The model under review builds one solid part; all positions refer to its coordinate system, in mm. A direction names the side the tool comes from. Give positions to 0.01 mm unless a question says otherwise; leave off trailing zeros. Order: outer loops, then holes, each group sorted by start corner. A loop starts at its lowest first (then second) coordinate and runs counter-clockwise, first axis right, second up. Notation, with made-up numbers: (22.5, 14.25) - (56.5, 14.25) arc R20 ccw to (56.5, 19.25) - close; hole circle Ø2 at (45, 70.5). An arc over 180 degrees is marked (long way). Put each result on its own line as item: value.
```python
from build123d import *

# Parameters (mm, degrees)
BOSS_EXTRUDE1_DEPTH = 2
BOSS_EXTRUDE2_DEPTH = 13
SKETCH3_R           = 1.55
CUT_EXTRUDE1_DEPTH  = 16


with BuildPart() as part:
    # Sketch1 → Boss-Extrude1 (new body)
    with BuildSketch(Plane.XY):
        with BuildLine():
            Line((-31.239860577, -6.933333333), (-36, -6.933333333))
            Line((-36, -6.933333333), (-36, 6.933333333))
            Line((-36, 6.933333333), (-31.239860577, 6.933333333))
            ThreePointArc((-31.239860577, 6.933333333), (0, 32), (31.239860577, 6.933333333))
            Line((31.239860577, 6.933333333), (36, 6.933333333))
            Line((36, 6.933333333), (36, -6.933333333))
            Line((36, -6.933333333), (31.239860577, -6.933333333))
            ThreePointArc((31.239860577, -6.933333333), (0, -32), (-31.239860577, -6.933333333))
        make_face()
    extrude(amount=BOSS_EXTRUDE1_DEPTH)

    # Sketch2 → Boss-Extrude2 (add)
    with BuildSketch(Plane.XY.offset(2)):
        with BuildLine():
            Line((-29.428567245, 12.568191195), (-27.589281792, 11.782679245))
            ThreePointArc((-27.589281792, 11.782679245), (0, 30), (27.589281792, 11.782679245))
            Line((27.589281792, 11.782679245), (29.428567245, 12.568191195))
            ThreePointArc((29.428567245, 12.568191195), (0, 32), (-29.428567245, 12.568191195))
        make_face()
        with BuildLine():
            Line((27.589281792, -11.782679245), (29.428567245, -12.568191195))
            ThreePointArc((29.428567245, -12.568191195), (0, -32), (-29.428567245, -12.568191195))
            Line((-29.428567245, -12.568191195), (-27.589281792, -11.782679245))
            ThreePointArc((-27.589281792, -11.782679245), (0, -30), (27.589281792, -11.782679245))
        make_face()
    extrude(amount=BOSS_EXTRUDE2_DEPTH)

    # Sketch3 → Cut-Extrude1 (cut, through all)
    with BuildSketch(Plane(origin=(0, 0, 0), x_dir=(-1, 0, 0), z_dir=(0, 0, -1))):
        with Locations((-33, 0)):
            Circle(SKETCH3_R)
        with Locations((33, 0)):
            Circle(SKETCH3_R)
    extrude(amount=-CUT_EXTRUDE1_DEPTH, mode=Mode.SUBTRACT)


solid = part.part
```
(1) Take a section at D-D, the plane y = 15.5. Write out the cut boundary in (x, z), then the cut area to 3 significant figures.
The answers:
outline: (-28, 0) - (28, 0) - (28, 15) - (25.69, 15) - (25.69, 2) - (-25.69, 2) - (-25.69, 15) - (-28, 15) - close
area: 172 mm^2
(2) Take a section at B-B, the plane x = -33. Write out the cut boundary in (y, z).
The answers:
outline: (-6.93, 0) - (-1.55, 0) - (-1.55, 2) - (-6.93, 2) - close; (1.55, 0) - (6.93, 0) - (6.93, 2) - (1.55, 2) - close
(3) The part is to be moulded in two halves that separate along Y. For faces 1 (the flat face through (1, 0, 2)), 2 (the flat face through (34, -6.933, 1)), 3 (the flat face through (-2, -30.1, 15)), say which applies: pulls with the +Y half, pulls with the -Y half, needs draft (parallel to the pull), parting line crosses it, or undercut.
The answers:
face 1: undercut
face 2: pulls with the -Y half
face 3: needs draft
(4) Take a section at C-C, the plane z = 6. Write out the cut boundary in (x, y).
The answers:
outline: (-29.43, -12.57) arc R32 ccw to (29.43, -12.57) - (27.59, -11.78) arc R30 cw to (-27.59, -11.78) - close; (-29.43, 12.57) - (-27.59, 11.78) arc R30 cw to (27.59, 11.78) - (29.43, 12.57) arc R32 ccw to start
(5) Wall thickness on L1, parallel to Y at x = 33, z = 0.5; L2, parallel to Y at x = -1, z = 11.5; L3, parallel to Z at x = -24.5, y = 16: over which ranges is each line inside the solid? List them lowest first.
The answers:
L1: -6.93 to -1.55, 1.55 to 6.93
L2: -31.98 to -29.98, 29.98 to 31.98
L3: 0 to 2
(6) Take a section at A-A, the plane y = 0. Write out the cut boundary in (x, z).
The answers:
outline: (-36, 0) - (-34.55, 0) - (-34.55, 2) - (-36, 2) - close; (-31.45, 0) - (31.45, 0) - (31.45, 2) - (-31.45, 2) - close; (34.55, 0) - (36, 0) - (36, 2) - (34.55, 2) - close
(7) For faces 4 (the flat face through (-28.52, -12.18, 8.41)), 5 (the flat face through (-34, 6.933, 1)), 6 (the flat face through (28.5, -12.17, 8.41)), 7 (the flat face through (-34, -6.933, 1)), 8 (the flat face through (34, 6.933, 1)), list the 3-axis set-ups (+Z, -Z, +X, -X, +Y, -Y) from which the entire face can be reached by the end or side of a thin tool; tool diameter is ignored.
The answers:
face 4: +Z, -X
face 5: +Z, -Z, -X, +Y
face 6: +Z, +X
face 7: +Z, -Z, -X, -Y
face 8: +Z, -Z, +X, +Y
(8) Clearance check with flat-ended pins moving along their axes: pin 1 Ø2 at (x, z) = (-34.5, 1) entering from -Y; pin 2 Ø2 at (x, z) = (-21, 3) entering from +Y; pin 3 Ø2 at (y, z) = (23, 4) entering from +X; pin 4 Ø1.9 at (x, y) = (33, 0) entering from +Z. State where each tip first meets the part, or that it passes through.
The answers:
pin 1: y = -6.93
pin 2: y = 24.98
pin 3: x = 23.24
pin 4: through
